Source: three-view drawing plus pictorial views. Frame: mm from the lowest corner of the part. A direction names the side the tool comes from. Give positions to 0.01 mm unless a question says otherwise; leave off trailing zeros. Loops run counter-clockwise (first coordinate to the right, second up) from the corner with the lowest first, then second, coordinate; pieces in that order, holes last. Notation, with made-up numbers: (39, 85.25) -> (69, 85.25) arc R8 ccw to (69, 95.25) -> close; hole circle Ø11 at (-7.5, 83.25). An arc over 180 degrees is marked (long way). Answer in a Markdown table with one row per item. Add a question column.
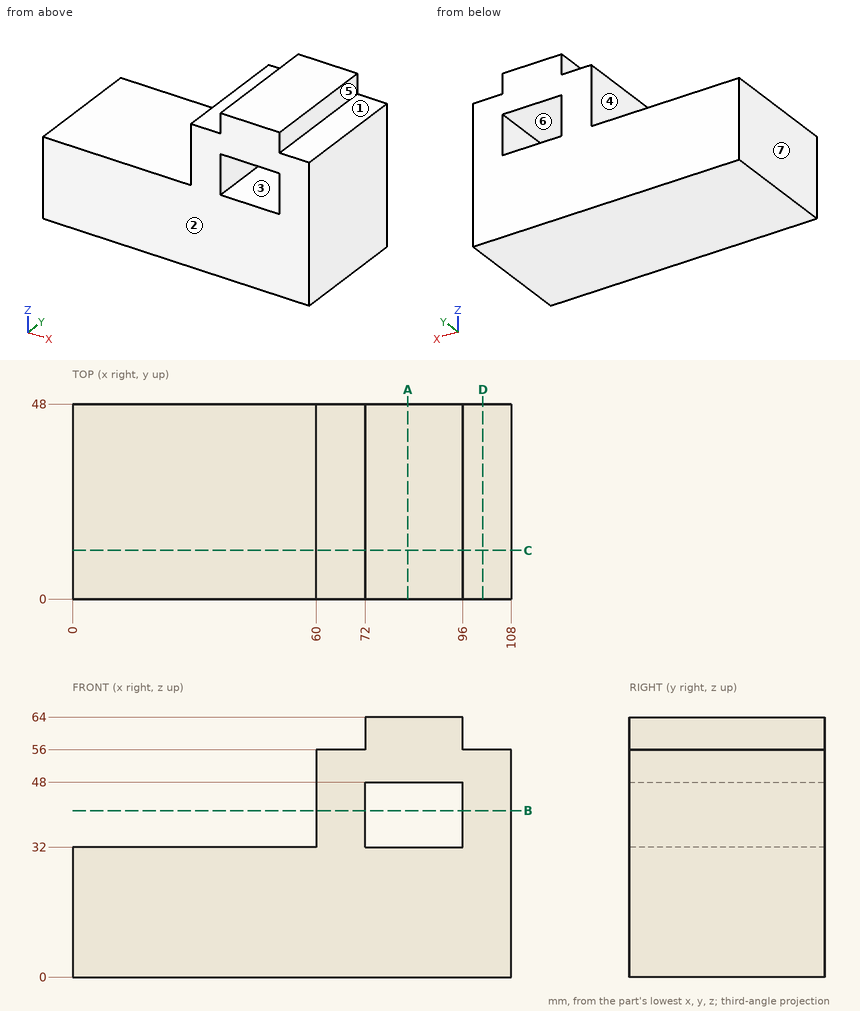
(1) Material intervals for line 1 along X through (y, z) = (5.5, 41.5); line 2 along Z through (x, y) = (77, 41.5); line 3 along Z through (x, y) = (50, 13.5), sorted ascending. Write a range as from..to.
(2) Cut plane D-D on x = 101. Return the cut outline in (y, z), then the cut area to 3 significant figures.
(3) Draft query along X for the marked faces 5, 6 and 7. Return one class per face: +X half, -X half, draft (parallel to the pull), parting line (faces both ways), or undercut.
(4) Pin query (flat end, axial travel): pin 1 Ø17.5 at (y, z) = (26, 42.5) entering from -X; pin 2 Ø24 at (x, y) = (32.5, 14) entering from +Z; pin 3 Ø3.5 at (x, y) = (65, 23.5) entering from +Z. Return the tip coordinate at first contact, or that it passes through.
(5) Reachability of the marked faces 1, 2, 3 and 4 from +Z, -Z, +X, -X, +Y, -Y: full face, straight path, thin tool, end or side. Return the list, or none.
(6) Cut plane C-C on y = 12. Return the cut outline in (x, z), then the cut area to 3 significant figures.
(7) Cut plane B-B on z = 41. Return the cut outline in (x, y), then the cut area to 3 significant figures.
(8) Cut plane A-A on x = 82.5. Return the cut outline in (y, z), then the cut area to 3 significant figures.
Answer list:
| question | item | result |
|---|---|---|
| 1 | line 1 | x = 60..72, 96..108 |
| 1 | line 2 | z = 0..32, 48..64 |
| 1 | line 3 | z = 0..32 |
| 2 | outline | (0, 0) -> (48, 0) -> (48, 56) -> (0, 56) -> close |
| 2 | area | 2,690 mm² |
| 3 | face 5 | +X half |
| 3 | face 6 | undercut |
| 3 | face 7 | -X half |
| 4 | pin 1 | stops at x = 60 |
| 4 | pin 2 | stops at z = 32 |
| 4 | pin 3 | stops at z = 56 |
| 5 | face 1 | +Z, +X, +Y, -Y |
| 5 | face 2 | +Z, -Z, +X, -X, -Y |
| 5 | face 3 | +Y, -Y |
| 5 | face 4 | +Z, -X, +Y, -Y |
| 6 | outline | (0, 0) -> (108, 0) -> (108, 56) -> (96, 56) -> (96, 64) -> (72, 64) -> (72, 56) -> (60, 56) -> (60, 32) -> (0, 32) -> close; hole (72, 32) -> (96, 32) -> (96, 48) -> (72, 48) -> close |
| 6 | area | 4,420 mm² |
| 7 | outline | (60, 0) -> (72, 0) -> (72, 48) -> (60, 48) -> close; (96, 0) -> (108, 0) -> (108, 48) -> (96, 48) -> close |
| 7 | area | 1,150 mm² |
| 8 | outline | (0, 0) -> (48, 0) -> (48, 32) -> (0, 32) -> close; (0, 48) -> (48, 48) -> (48, 64) -> (0, 64) -> close |
| 8 | area | 2,300 mm² |
